Job drawing, mm, ordinate dimensions from the low corner. One solid piece. Round coordinates to 2 decimals unless told otherwise and drop trailing zeros. Write each loop counter-clockwise with the first axis right and the second up, starting at its lowest first coordinate (ties: lowest second). Pieces come first, ordered by that corner, then holes. Notation, with made-up numbers: (10, 62.5) -> (21, 62.5) arc R17 cw to (21, 71.5) -> close; hole circle Ø9 at (59, 82). An arc over 180 degrees is marked (long way). Use CSV: the item, a comma, the result in double quotes. Start each with the question number.
(1) Drop flat-ended pins along their axis: pin 1 (7 mm diameter, centred on x = 9, z = 12, fed in from +Y); pin 2 (8 mm diameter, centred on x = 20.5, y = 10.5, fed in from -Z); pin 3 (3 mm diameter, centred on y = 35.5, z = 17, fed in from -X). Give the stop position or say it passes through.
(2) Saw through at B-B (z = 12.5). Give the cut face in (x, y).
(3) Saw through at A-A (x = 6). Give the cut face in (y, z), plus the area to 3 significant figures.
(4) Probe line 1 (Y direction, x = 15.25, z = 20.5); line 2 (X direction, y = 64.75, z = 12.5); line 3 (X direction, y = 12, z = 12.25). List the from-to ranges inside material, lowest first. Write a range as [from, to].
(5) Saw through at D-D (z = 6.25). Give the cut face in (x, y), plus the area to 3 significant figures.
(6) Saw through at C-C (x = 12.5). Give the cut face in (y, z), plus the area to 3 significant figures.
(7) Two-plate mould, pull along Y, no slides. Class the marked faces 1, 2, 3 and 4: released by +Y, released by -Y, zero draft, split by the parting line, or undercut.
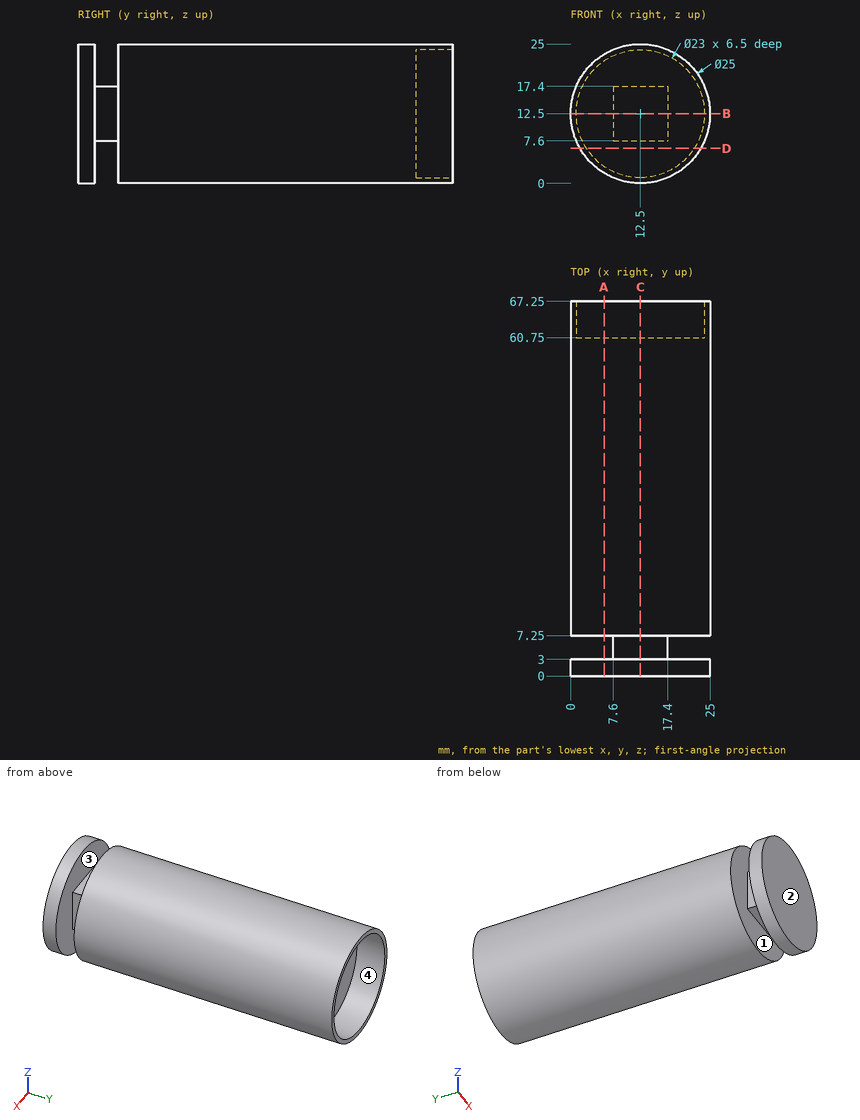
Answers:
1,pin 1,"stops at y = 60.75"
1,pin 2,"stops at z = 0.66"
1,pin 3,"stops at x = 0.37"
2,outline,"(0, 0) -> (25, 0) -> (25, 3) -> (17.4, 3) -> (17.4, 7.25) -> (25, 7.25) -> (25, 67.25) -> (24, 67.25) -> (24, 60.75) -> (1, 60.75) -> (1, 67.25) -> (0, 67.25) -> (0, 7.25) -> (7.6, 7.25) -> (7.6, 3) -> (0, 3) -> close"
3,outline,"(0, 1.82) -> (3, 1.82) -> (3, 23.18) -> (0, 23.18) -> close; (7.25, 1.82) -> (67.25, 1.82) -> (67.25, 3.01) -> (60.75, 3.01) -> (60.75, 21.99) -> (67.25, 21.99) -> (67.25, 23.18) -> (7.25, 23.18) -> close"
3,area,"1,220 mm²"
4,line 1,"y = [0, 3], [7.25, 60.75]"
4,line 2,"x = [0, 1], [24, 25]"
4,line 3,"x = [0, 25]"
5,outline,"(1.67, 0) -> (23.33, 0) -> (23.33, 3) -> (1.67, 3) -> close; (1.67, 7.25) -> (23.33, 7.25) -> (23.33, 67.25) -> (22.15, 67.25) -> (22.15, 60.75) -> (2.85, 60.75) -> (2.85, 67.25) -> (1.67, 67.25) -> close"
5,area,"1,240 mm²"
6,outline,"(0, 0) -> (3, 0) -> (3, 7.6) -> (7.25, 7.6) -> (7.25, 0) -> (67.25, 0) -> (67.25, 1) -> (60.75, 1) -> (60.75, 24) -> (67.25, 24) -> (67.25, 25) -> (7.25, 25) -> (7.25, 17.4) -> (3, 17.4) -> (3, 25) -> (0, 25) -> close"
6,area,"1,470 mm²"
7,face 1,"undercut"
7,face 2,"released by -Y"
7,face 3,"undercut"
7,face 4,"zero draft"
